The model under review builds one solid part; all positions refer to its coordinate system, in mm. A direction names the side the tool comes from. Give positions to 0.01 mm unless a question says otherwise; leave off trailing zeros. Loops run counter-clockwise (first coordinate to the right, second up) from the corner with the lowest first, then second, coordinate; pieces in that order, holes last. Notation, with made-up numbers: (-23, -24) -> (29, -24) arc R23 ccw to (29, -7) -> close; hole circle Ø7 at (19.25, 20.25). An arc over 180 degrees is marked (long way). Write each question's results on one line, items separated by ' | '. Start each with the question number.
Q1. We need section B-B (x = 16.8). Write out the cut boundary in (y, z), plus the area to 3 significant figures.
Q2. We need section D-D (x = 3). Write out the cut boundary in (y, z).
Q3. We need section C-C (z = -7.5). Write out the cut boundary in (x, y).
Q4. Wall thickness on L1, parallel to X at y = 6.25, z = -11.5; L2, parallel to Y at x = 48, z = -3; L3, parallel to Z at x = 17, y = 10: over which ranges is each line inside the solid? List them lowest first. Write a range as [from, to].
Q5. Machinability: for faces 4 (the face through (61.8, 9.5, -10.5)), 5 (the face through (54.7, 10, -11)), 6 (the face through (68.5, 8.4, -2.9)), which of the approach directions +Z, -Z, +X, -X, +Y, -Y give a long, thin tool a straight path to every point of the face, cutting with its end or side? Answer none if there is none.
Q6. Mouldability with a two-part tool opening along Z and no side actions: class faces 1 (the face through (7, 9.5, -10.5)), 2 (the face through (7, 12, -16)), 3 (the face through (53.49, 23.381, -13.024)) as released by +Z, released by -Z, zero draft, split by the parting line, or undercut.
Q7. We need section A-A (y = 14.25). Write out the cut boundary in (x, z), plus the area to 3 significant figures.
Q8. Insertion check: pin 1 Ø8 at (y, z) = (11.5, -15.5) entering from +X; pin 2 Ø1 at (y, z) = (10.5, -2.5) entering from -X; pin 3 Ø4 at (x, y) = (16.5, 11) entering from -Z; pin 4 Ø12 at (x, y) = (27.5, 24) entering from +Z. Each pin has a flat end and moves straight along its axis. Give the tip position at first contact, or say it passes through.
from build123d import *
from OCP.BRepFilletAPI import BRepFilletAPI_MakeChamfer

# Parameters (mm, degrees)
SKETCH_1_W             = 69
SKETCH_1_H             = 20
EXTRUDE_1_DEPTH        = 3
FILLET_1_R             = 1
SKETCH_3_W             = 12.25
SKETCH_3_H             = 11.5
SKETCH_3_W_2           = 17.5
EXTRUDE_2_DEPTH        = 6
SKETCH_4_W             = 5
SKETCH_4_H             = 10.6
EXTRUDE_3_DEPTH        = 9
SKETCH_5_R             = 2.4
EXTRUDE_4_DEPTH        = 17
CHAMFER_1_SIZE         = 4
CHAMFER_1_SIZE2        = 5
EXTRUDE_5_DEPTH        = 4.8
MIRROR_START           = 3
MIRROR_1_OUTLINE_W     = 69
MIRROR_1_OUTLINE_H     = 20
MIRROR_1_DEPTH         = 3
MIRROR_START_2         = 6
MIRROR_1_2_OUTLINE_W   = 5
MIRROR_1_2_OUTLINE_H   = 10.6
MIRROR_1_2_DEPTH       = 9
MIRROR_START_3         = 15
MIRROR_1_3_OUTLINE_R   = 2.4
MIRROR_1_3_DEPTH       = 17
MIRROR_1_4_OUTLINE_W   = 12.25
MIRROR_1_4_OUTLINE_H   = 11.5
MIRROR_1_4_OUTLINE_W_2 = 17.5
MIRROR_1_4_DEPTH       = 1
MIRROR_START_4         = 6.49884
MIRROR_1_5_DEPTH       = 4.30116
MIRROR_START_5         = 25.75
MIRROR_1_6_DEPTH       = 17.5
MIRROR_START_6         = 1
MIRROR_1_7_DEPTH       = 12.25
MIRROR_START_7         = 55.75
MIRROR_1_8_DEPTH       = 12.25
SKETCH_7_W             = 69
SKETCH_7_H             = 20
CUT_EXTRUDE_1_DEPTH    = 78.472575793


with BuildPart() as part:
    # ｽｹｯﾁ1 → ﾎﾞｽ - 押し出し1 (new body)
    with BuildSketch(Plane(origin=(0, 0, 0), x_dir=(1, 0, 0), z_dir=(0, 1, 0))):
        with Locations((34.5, 10)):
            Rectangle(SKETCH_1_W, SKETCH_1_H)
    extrude(amount=EXTRUDE_1_DEPTH)

    # ﾌｨﾚｯﾄ1
    fillet_1_edges = [part.edges().sort_by_distance(p)[0] for p in [
        (0, 1.5, -20),
        (69, 1.5, -20),
        (69, 1.5, 0),
        (0, 1.5, 0),
    ]]
    fillet(fillet_1_edges, radius=FILLET_1_R)

    # ｽｹｯﾁ3 → ﾎﾞｽ - 押し出し2 (add)
    with BuildSketch(Plane.XZ):
        with Locations((7.125, -14.25)):
            Rectangle(SKETCH_3_W, SKETCH_3_H)
        with Locations((34.5, -14.25)):
            Rectangle(SKETCH_3_W_2, SKETCH_3_H)
        with Locations((61.875, -14.25)):
            Rectangle(SKETCH_3_W, SKETCH_3_H)
    extrude(amount=EXTRUDE_2_DEPTH)

    # ｽｹｯﾁ4 → ﾎﾞｽ - 押し出し3 (add)
    with BuildSketch(Plane.XZ):
        with Locations((52.2, -11)):
            Rectangle(SKETCH_4_W, SKETCH_4_H)
        with Locations((16.8, -11)):
            Rectangle(SKETCH_4_W, SKETCH_4_H)
    extrude(amount=EXTRUDE_3_DEPTH)

    # ｽｹｯﾁ5 → ﾎﾞｽ - 押し出し4 (add)
    with BuildSketch(Plane.XZ.offset(9)):
        with Locations(Location((16.8, -11, 0), (0, 0, 270))):
            Circle(SKETCH_5_R)
        with Locations(Location((52.2, -11, 0), (0, 0, 90))):
            Circle(SKETCH_5_R)
    extrude(amount=EXTRUDE_4_DEPTH)

    # 面取り1: one chamfer whose edges measure the first distance from different faces: ONE call of the kernel's chamfer builder (chamfer() names one face for all edges)
    chamfer_1_edges_1 = [part.edges().sort_by_distance(p)[0] for p in [
        (7.125, -6, -8.5),
    ]]
    chamfer_1_side_1 = [part.faces().sort_by_distance(p)[0] for p in [
        (7.125, -3, -8.5),
    ]]
    chamfer_1_edges_2 = [part.edges().sort_by_distance(p)[0] for p in [
        (34.5, -6, -8.5),
    ]]
    chamfer_1_side_2 = [part.faces().sort_by_distance(p)[0] for p in [
        (34.5, -3, -8.5),
    ]]
    chamfer_1_edges_3 = [part.edges().sort_by_distance(p)[0] for p in [
        (61.875, -6, -8.5),
    ]]
    chamfer_1_side_3 = [part.faces().sort_by_distance(p)[0] for p in [
        (61.875, -3, -8.5),
    ]]
    chamfer_1 = BRepFilletAPI_MakeChamfer(part.part.solid().wrapped)
    for e in chamfer_1_edges_1:
        chamfer_1.Add(CHAMFER_1_SIZE, CHAMFER_1_SIZE2, e.wrapped, chamfer_1_side_1[0].wrapped)  # the first distance lies on this face
    for e in chamfer_1_edges_2:
        chamfer_1.Add(CHAMFER_1_SIZE, CHAMFER_1_SIZE2, e.wrapped, chamfer_1_side_2[0].wrapped)  # the first distance lies on this face
    for e in chamfer_1_edges_3:
        chamfer_1.Add(CHAMFER_1_SIZE, CHAMFER_1_SIZE2, e.wrapped, chamfer_1_side_3[0].wrapped)  # the first distance lies on this face
    add(Compound.cast(chamfer_1.Shape()), mode=Mode.REPLACE)

    # ｽｹｯﾁ6 → ﾎﾞｽ - 押し出し5 (add)
    with BuildSketch(Plane.XZ):
        with BuildLine():
            Line((4.4, -5.071231518), (4.4, -0.928768482))
            ThreePointArc((4.4, -0.928768482), (0.5, -3), (4.4, -5.071231518))
        make_face()
        with BuildLine():
            ThreePointArc((68.5, -3), (67.17260394, -0.792059783), (64.6, -0.928768482))
            Line((64.6, -0.928768482), (64.6, -5.071231518))
            ThreePointArc((64.6, -5.071231518), (67.17260394, -5.207940217), (68.5, -3))
        make_face()
    extrude(amount=EXTRUDE_5_DEPTH)

    # ﾐﾗｰ1: read off the stored shape, not the designer's step
    # ﾐﾗｰ1 outline → ﾐﾗｰ1 (add)
    with BuildSketch(Plane(origin=(0, 0, 0), x_dir=(1, 0, 0), z_dir=(0, 1, 0)).offset(MIRROR_START)):
        with Locations((34.5, 10)):
            Rectangle(MIRROR_1_OUTLINE_W, MIRROR_1_OUTLINE_H)
    extrude(amount=MIRROR_1_DEPTH)

    # Mirror 1 2 outline → Mirror 1 2 (add)
    with BuildSketch(Plane(origin=(0, 0, 0), x_dir=(1, 0, 0), z_dir=(0, 1, 0)).offset(MIRROR_START_2)):
        with Locations((52.2, 11)):
            Rectangle(MIRROR_1_2_OUTLINE_W, MIRROR_1_2_OUTLINE_H)
        with Locations((16.8, 11)):
            Rectangle(MIRROR_1_2_OUTLINE_W, MIRROR_1_2_OUTLINE_H)
    extrude(amount=MIRROR_1_2_DEPTH)

    # Mirror 1 3 outline → Mirror 1 3 (add)
    with BuildSketch(Plane(origin=(0, 0, 0), x_dir=(1, 0, 0), z_dir=(0, 1, 0)).offset(MIRROR_START_3)):
        with Locations((16.8, 11)):
            Circle(MIRROR_1_3_OUTLINE_R)
        with Locations((52.2, 11)):
            Circle(MIRROR_1_3_OUTLINE_R)
    extrude(amount=MIRROR_1_3_DEPTH)

    # Mirror 1 4 outline → Mirror 1 4 (add)
    with BuildSketch(Plane(origin=(0, 0, 0), x_dir=(1, 0, 0), z_dir=(0, 1, 0)).offset(MIRROR_START_2)):
        with Locations((7.125, 14.25)):
            Rectangle(MIRROR_1_4_OUTLINE_W, MIRROR_1_4_OUTLINE_H)
        with Locations((61.875, 14.25)):
            Rectangle(MIRROR_1_4_OUTLINE_W, MIRROR_1_4_OUTLINE_H)
        with Locations((34.5, 14.25)):
            Rectangle(MIRROR_1_4_OUTLINE_W_2, MIRROR_1_4_OUTLINE_H)
        with BuildLine():
            ThreePointArc((4.4, 5.071231518), (0.5, 3), (4.4, 0.928768482))
            Line((4.4, 0.928768482), (4.4, 5.071231518))
        make_face()
        with BuildLine():
            ThreePointArc((64.6, 0.928768482), (68.5, 3), (64.6, 5.071231518))
            Line((64.6, 5.071231518), (64.6, 0.928768482))
        make_face()
    extrude(amount=MIRROR_1_4_DEPTH)

    # Mirror 1 5 outline → Mirror 1 5 (add)
    with BuildSketch(Plane(origin=(0, 0, 0), x_dir=(1, 0, 0), z_dir=(0, 1, 0)).offset(MIRROR_START_4)):
        with BuildLine():
            ThreePointArc((4.4, 5.071231518), (0.5, 3), (4.4, 0.928768482))
            Line((4.4, 0.928768482), (4.4, 5.071231518))
        make_face()
        with BuildLine():
            ThreePointArc((64.6, 0.928768482), (68.5, 3), (64.6, 5.071231518))
            Line((64.6, 5.071231518), (64.6, 0.928768482))
        make_face()
    extrude(amount=MIRROR_1_5_DEPTH)

    # Mirror 1 6 outline → Mirror 1 6 (add)
    with BuildSketch(Plane.YZ.offset(MIRROR_START_5)):
        Polygon((7, -20), (12, -20), (12, -12.5), (7, -8.5), align=None)
    extrude(amount=MIRROR_1_6_DEPTH)

    # Mirror 1 7 outline → Mirror 1 7 (add)
    with BuildSketch(Plane.YZ.offset(MIRROR_START_6)):
        Polygon((7, -20), (12, -20), (12, -12.5), (7, -8.5), align=None)
    extrude(amount=MIRROR_1_7_DEPTH)

    # Mirror 1 8 outline → Mirror 1 8 (add)
    with BuildSketch(Plane.YZ.offset(MIRROR_START_7)):
        Polygon((7, -20), (12, -20), (12, -12.5), (7, -8.5), align=None)
    extrude(amount=MIRROR_1_8_DEPTH)

    # ｽｹｯﾁ7 → ｶｯﾄ - 押し出し1 (cut, through all)
    with BuildSketch(Plane.XZ.offset(-3)):
        with Locations((34.5, -10)):
            Rectangle(SKETCH_7_W, SKETCH_7_H)
    extrude(amount=CUT_EXTRUDE_1_DEPTH, mode=Mode.SUBTRACT)


solid = part.part
Output:
1) outline: (3, -20) -> (6, -20) -> (6, -16.3) -> (15, -16.3) -> (15, -13.4) -> (32, -13.4) -> (32, -8.6) -> (15, -8.6) -> (15, -5.7) -> (6, -5.7) -> (6, 0) -> (3, 0) -> close | area: 237 mm2
2) outline: (3, -20) -> (12, -20) -> (12, -12.5) -> (7, -8.5) -> (6, -8.5) -> (6, -5.5) -> (10.8, -5.5) -> (10.8, -0.5) -> (6, -0.5) -> (6, 0) -> (3, 0) -> close
3) outline: (0, 3) -> (69, 3) -> (69, 6) -> (54.7, 6) -> (54.7, 15) -> (49.7, 15) -> (49.7, 6) -> (19.3, 6) -> (19.3, 15) -> (14.3, 15) -> (14.3, 6) -> (0, 6) -> close
4) L1: [1, 13.25], [14.3, 19.3], [25.75, 43.25], [49.7, 54.7], [55.75, 68] | L2: [3, 6] | L3: [-16.3, -5.7]
5) face 4: +X, +Y | face 5: +Z, -Z, +Y | face 6: +Y
6) face 1: undercut | face 2: zero draft | face 3: split by the parting line
7) outline: (14.3, -16.3) -> (19.3, -16.3) -> (19.3, -5.7) -> (14.3, -5.7) -> close; (49.7, -16.3) -> (54.7, -16.3) -> (54.7, -5.7) -> (49.7, -5.7) -> close | area: 106 mm2
8) pin 1: x = 68 | pin 2: x = 0.5 | pin 3: z = -16.3 | pin 4: through
